Here's how the part is built. I have some questions about the finished solid (model axes, mm). Give positions to 0.01 mm unless a question says otherwise; leave off trailing zeros. Use a Markdown table: item, result.
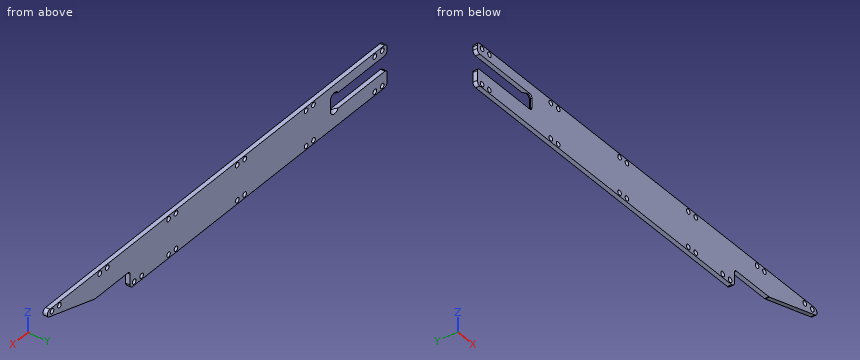
```python
from build123d import *

# Parameters (mm, degrees)
BOSS_EXTRUDE1_DEPTH  = 3
M3_CLEARANCE_HOLE1_D = 3.4
CUT_EXTRUDE5_DEPTH   = 10
FILLET3_R            = 2
CHAMFER1_SIZE        = 2
SKETCH30_R           = 1.7
BOSS_EXTRUDE3_DEPTH  = 3
FILLET4_R            = 2.5


with BuildPart() as part:
    # Sketch1 → Boss-Extrude1 (new body)
    with BuildSketch(Plane(origin=(0, 0, 0), x_dir=(1, 0, 0), z_dir=(0, 1, 0))):
        with BuildLine():
            Line((-135.5, 14.75), (135.5, 14.75))
            ThreePointArc((135.5, 14.75), (137.267766953, 14.017766953), (138, 12.25))
            Line((138, 12.25), (138, -12.25))
            ThreePointArc((138, -12.25), (137.267766953, -14.017766953), (135.5, -14.75))
            Line((135.5, -14.75), (-135.5, -14.75))
            ThreePointArc((-135.5, -14.75), (-137.267766953, -14.017766953), (-138, -12.25))
            Line((-138, -12.25), (-138, 12.25))
            ThreePointArc((-138, 12.25), (-137.267766953, 14.017766953), (-135.5, 14.75))
        make_face()
    extrude(amount=BOSS_EXTRUDE1_DEPTH)

    # M3 Clearance Hole1 (through all)
    with Locations(Plane.XZ):
        with Locations((-133.5, 12.25), (-126.5, 12.25), (-133.5, -12.25), (-126.5, -12.25), (-68.5, 12.25), (-61.5, 12.25), (-68.5, -12.25), (-61.5, -12.25), (-3.5, 12.25), (3.5, 12.25), (-3.5, -12.25), (3.5, -12.25), (61.5, 12.25), (68.5, 12.25), (61.5, -12.25), (68.5, -12.25), (126.5, 12.25), (133.5, 12.25), (126.5, -12.25), (133.5, -12.25), (94, -12.25), (101, -12.25)):
            Hole(M3_CLEARANCE_HOLE1_D / 2)

    # Sketch29 → Cut-Extrude5 (cut)
    with BuildSketch(Plane.XZ):
        with BuildLine():
            Line((105, -14.75), (105, -4.75))
            ThreePointArc((105, -4.75), (105.585786438, -3.335786438), (107, -2.75))
            Line((107, -2.75), (138, -2.75))
            Line((138, -2.75), (138, -14.75))
            Line((138, -14.75), (105, -14.75))
        make_face()
        with BuildLine():
            Line((-86.41637679, 5.3456), (-86.41637679, -1.4522))
            ThreePointArc((-86.41637679, -1.4522), (-87.002163227, -2.866413562), (-88.41637679, -3.4522))
            Line((-88.41637679, -3.4522), (-138, -3.4522))
            Line((-138, -3.4522), (-138, 9.8456))
            ThreePointArc((-138, 9.8456), (-137.267766953, 8.077833047), (-135.5, 7.3456))
            Line((-135.5, 7.3456), (-88.41637679, 7.3456))
            ThreePointArc((-88.41637679, 7.3456), (-87.002163227, 6.759813562), (-86.41637679, 5.3456))
        make_face()
    extrude(amount=-CUT_EXTRUDE5_DEPTH, mode=Mode.SUBTRACT)

    # Fillet3
    fillet3_edges = [part.edges().sort_by_distance(p)[0] for p in [
        (-138, 1.5, -3.4522),
    ]]
    fillet(fillet3_edges, radius=FILLET3_R)

    # Chamfer1
    # the kernel refuses this chamfer: 2 mm, written as the material it takes off along each edge
    with BuildSketch(Plane(origin=(-88.41637679, 3, 5.3456), x_dir=(1, 0, 0), z_dir=(0, 0, -1))) as chamfer1_piece_1:
        Polygon((2, CHAMFER1_SIZE), (2 + CHAMFER1_SIZE, 0), (2, 0), align=None)
    revolve(axis=Axis((-88.41637679, 3, 5.3456), (0, -1, 0)), revolution_arc=237.405771779, mode=Mode.SUBTRACT)
    with BuildSketch(Plane(origin=(-86.41637679, 3, 5.3456), x_dir=(-0.027495876610589075, -0.9996219169112968, 0), z_dir=(0, 0, -1))) as chamfer1_piece_2:
        Polygon((CHAMFER1_SIZE * 0.999621916911, -CHAMFER1_SIZE * 0.0274958766106), (-CHAMFER1_SIZE * 0.0274958766106, -CHAMFER1_SIZE * 0.999621916911), (0, 0), align=None)
    extrude(amount=6.7978, mode=Mode.SUBTRACT)
    with BuildSketch(Plane(origin=(-88.41637679, 3, -1.4522), x_dir=(-0.5386859165215122, 0, 0.842506666645065), z_dir=(0.842506666645065, 0, 0.5386859165215122))) as chamfer1_piece_3:
        Polygon((2, CHAMFER1_SIZE), (2 + CHAMFER1_SIZE, 0), (2, 0), align=None)
    revolve(axis=Axis((-88.41637679, 3, -1.4522), (0, -1, 0)), revolution_arc=237.405771779, mode=Mode.SUBTRACT)

    # Sketch30 → Boss-Extrude3 (add)
    with BuildSketch(Plane.XZ):
        with BuildLine():
            Line((138, -2.75), (181.384803676, 9.849187775))
            ThreePointArc((181.384803676, 9.849187775), (183.162673325, 12.602114639), (180.687594482, 14.75))
            Line((180.687594482, 14.75), (135.5, 14.75))
            ThreePointArc((135.5, 14.75), (137.267766953, 14.017766953), (138, 12.25))
            Line((138, 12.25), (138, -2.75))
        make_face()
        with Locations(Location((171.687594482, 12.25, 0), (0, 0, 270))):
            Circle(SKETCH30_R, mode=Mode.SUBTRACT)
        with Locations(Location((178.687594482, 12.25, 0), (0, 0, 270))):
            Circle(SKETCH30_R, mode=Mode.SUBTRACT)
    extrude(amount=-BOSS_EXTRUDE3_DEPTH)

    # Fillet4
    fillet4_edges = [part.edges().sort_by_distance(p)[0] for p in [
        (105, 1.5, -14.75),
        (138, 1.5, -2.75),
    ]]
    fillet(fillet4_edges, radius=FILLET4_R)


solid = part.part
```
Item 1: If we section it at A-A, the plane y = 2.5: Count the separate pieces of the cut face and the enclosed holes in it, plus the area to 3 significant figures.
Values:
| item | result |
|---|---|
| separate pieces | 1 |
| enclosed holes | 22 |
| area | 7,450 mm2 |
Item 2: I need wall thicknesses on line 1 along Z through (x, y) = (-126.5, 0.75); line 2 along Z through (x, y) = (68.5, 2); line 3 along Z through (x, y) = (-118.5, 1.6). Which ranges of each line are inside material? Lowest first, please. Write a range as [from, to].
Values:
| item | result |
|---|---|
| line 1 | z = [-14.75, -13.95], [-10.55, -3.45], [7.35, 10.55], [13.95, 14.75] |
| line 2 | z = [-14.75, -13.95], [-10.55, 10.55], [13.95, 14.75] |
| line 3 | z = [-14.75, -3.45], [7.35, 14.75] |
Item 3: Will these pins go through, and if not, where does the flat tip stop? pin 1 Ø3 at (x, z) = (-77, -8.5) entering from -Y; pin 2 Ø1.5 at (y, z) = (1, -6.5) entering from +X; pin 3 Ø1.5 at (x, y) = (115, 2) entering from -Z.
Values:
| item | result |
|---|---|
| pin 1 | stops at y = 0 |
| pin 2 | stops at x = 105 |
| pin 3 | stops at z = -2.75 |
